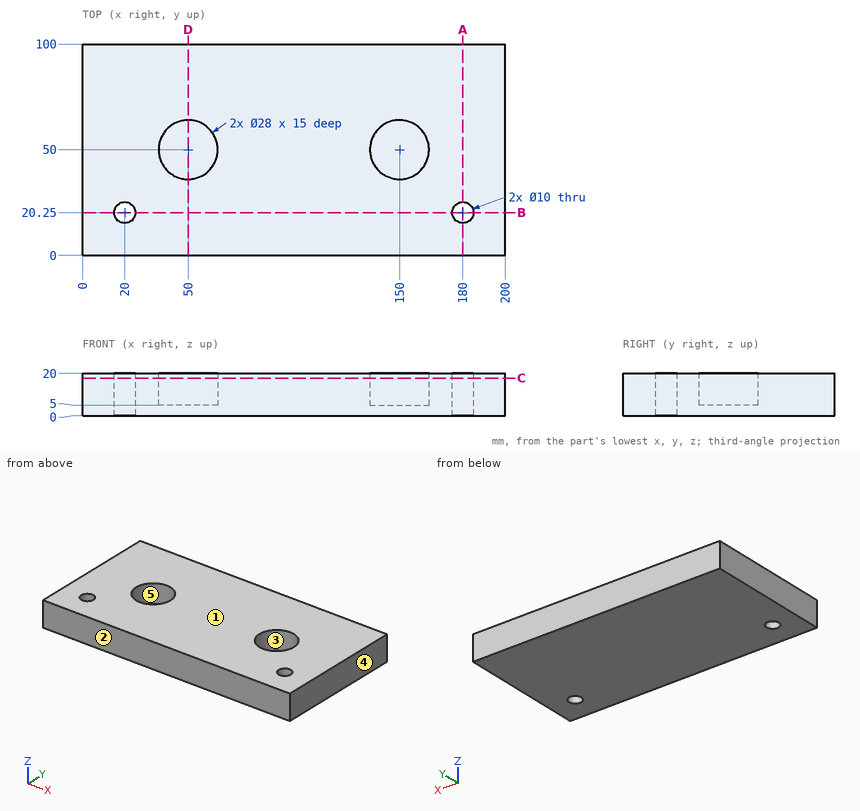
Print and shaded views of the part. All mm, measured from the part's lowest x, y and z. A direction names the side the tool comes from. Give positions to 0.01 mm unless a question says otherwise; leave off trailing zeros. Loops run counter-clockwise (first coordinate to the right, second up) from the corner with the lowest first, then second, coordinate; pieces in that order, holes last. Notation, with made-up numbers: M 68.25,21.25 L 99.25,21.25 A24 cw 99.25,57.25 Z; hole C -5.75,-37 d11. An arc over 180 degrees is marked long. Write each question's results on one line, items separated by ' | '.
Q1. Band-saw the part on C-C on z = 17.75. Write the cut outline in (x, y).
Geometry check:
outline: M 0,0 L 200,0 L 200,100 L 0,100 Z; hole C 20,20.25 d10; hole C 50,50 d28; hole C 150,50 d28; hole C 180,20.25 d10
Q2. Mould opens along Y. For the marked faces 1, 2 and 3 say: pulls with the +Y half, pulls with the -Y half, needs draft (parallel to the pull), parting line crosses it, or undercut.
Geometry check:
face 1: needs draft | face 2: pulls with the -Y half | face 3: undercut
Q3. Band-saw the part on B-B on y = 20.25. Write the cut outline in (x, z), and give its area (3 significant figures).
Geometry check:
outline: M 0,0 L 15,0 L 15,20 L 0,20 Z; M 25,0 L 175,0 L 175,20 L 25,20 Z; M 185,0 L 200,0 L 200,20 L 185,20 Z | area: 3,600 mm²
Q4. Flat gauge pin, fed straight in: P1, Ø14, axis at x = 150, y = 47, coming from the +Z side. Where does the tip first touch, or does it go through?
Geometry check:
P1: stops at z = 5
Q5. Which spindle directions (+Z, -Z, +X, -X, +Y, -Y) get a long thin tool onto all of the face, cutting with end or side? Do the marked faces 4 and 5. Say none if no direction does.
Geometry check:
face 4: +Z, -Z, +X, +Y, -Y | face 5: +Z
Q6. Band-saw the part on D-D on x = 50. Write the cut outline in (y, z).
Geometry check:
outline: M 0,0 L 100,0 L 100,20 L 64,20 L 64,5 L 36,5 L 36,20 L 0,20 Z
Q7. Probe probe 1 along Y at (x, z) = (180, 14.75); probe 2 along X at (y, z) = (18.5, 10.5); probe 3 along X at (y, z) = (18, 14.5). List the from-to ranges inside material, lowest first.
Geometry check:
probe 1: y = 0 to 15.25, 25.25 to 100 | probe 2: x = 0 to 15.32, 24.68 to 175.32, 184.68 to 200 | probe 3: x = 0 to 15.53, 24.47 to 175.53, 184.47 to 200
Q8. Band-saw the part on A-A on x = 180. Write the cut outline in (y, z), and give its area (3 significant figures).
Geometry check:
outline: M 0,0 L 15.25,0 L 15.25,20 L 0,20 Z; M 25.25,0 L 100,0 L 100,20 L 25.25,20 Z | area: 1,800 mm²
